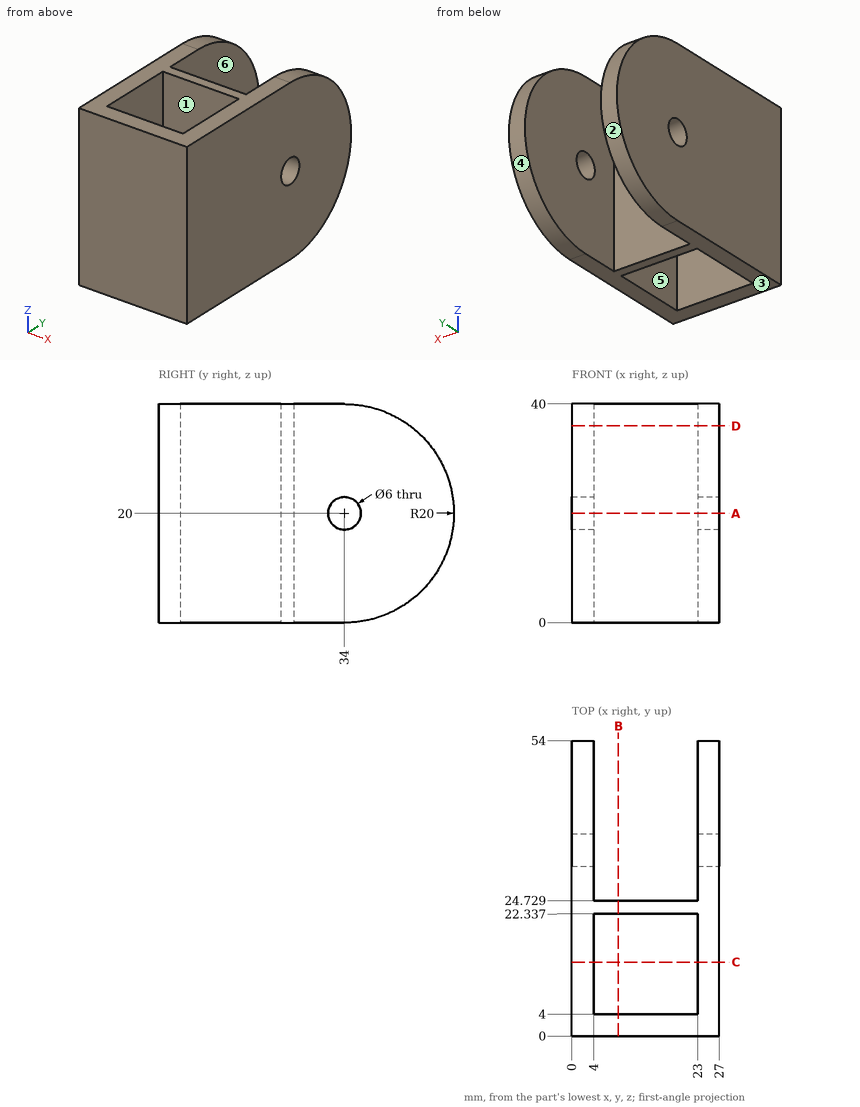
Can you work these out from the drawing? Everything is in mm from the part's minimum corner. A direction names the side the tool comes from. Round coordinates to 2 decimals unless told otherwise and drop trailing zeros. Loops run counter-clockwise (first coordinate to the right, second up) from the corner with the lowest first, then second, coordinate; pieces in that order, holes last. Notation, with made-up numbers: M 53,60 L 83,60 A29 ccw 83,80 Z; hole C 58.25,72 d3. An arc over 180 degrees is marked long. Write item = value, one per line.
1. Will these pins go through, and if not, where does the flat tip stop? P1, Ø10, axis at x = 6.5, z = 6.5, coming from the +Y side (1 decimal); P2, Ø8, axis at x = 7.5, z = 17, coming from the -Y side; P3, Ø5.5, axis at x = 12.5, z = 19, coming from the +Y side.
Results below:
P1 = 51.8
P2 = 0
P3 = 24.73
2. I want a section at C-C, the plane y = 13.5. Write out the boundary of the cut face in (x, z).
Results below:
outline = M 0,0 L 4,0 L 4,40 L 0,40 Z; M 23,0 L 27,0 L 27,40 L 23,40 Z
3. Which directions (+Z, -Z, +X, -X, +Y, -Y) give clear straight access to the entire face, cutting with the end or side of a thin tool? Please do the marked faces 4, 5 and 6.
Results below:
face_4 = +X, -X, +Y
face_5 = +Z, -Z
face_6 = +Z, -Z, +Y
4. I want a section at D-D, the plane z = 36. Write out the boundary of the cut face in (x, y).
Results below:
outline = M 0,0 L 27,0 L 27,46 L 23,46 L 23,24.73 L 4,24.73 L 4,46 L 0,46 Z; hole M 4,4 L 23,4 L 23,22.34 L 4,22.34 Z
5. I need wall thicknesses on probe 1 along Y at (x, z) = (22.25, 17); probe 2 along X at (y, z) = (15.5, 7.5); probe 3 along Z at (x, y) = (24.9, 34). Which ranges of each line are inside material? Lowest first, please.
Results below:
probe_1 = 0 to 4, 22.34 to 24.73
probe_2 = 0 to 4, 23 to 27
probe_3 = 0 to 17, 23 to 40
6. I want a section at B-B, the plane x = 8.5. Write out the boundary of the cut face in (y, z), and give its area (3 significant figures).
Results below:
outline = M 0,0 L 4,0 L 4,40 L 0,40 Z; M 22.34,0 L 24.73,0 L 24.73,40 L 22.34,40 Z
area = 256 mm²
7. Thinking about a two-plate mould opening in Y: for the marked faces 1, 2 and 3, which applies, +Y half, -Y half, draft (parallel to the pull), parting line (faces both ways), or undercut?
Results below:
face_1 = undercut
face_2 = +Y half
face_3 = draft
8. I want a section at A-A, the plane z = 20. Write out the boundary of the cut face in (x, y).
Results below:
outline = M 0,0 L 27,0 L 27,31 L 23,31 L 23,24.73 L 4,24.73 L 4,31 L 0,31 Z; M 0,37 L 4,37 L 4,54 L 0,54 Z; M 23,37 L 27,37 L 27,54 L 23,54 Z; hole M 4,4 L 23,4 L 23,22.34 L 4,22.34 Z
